Design review of the part built by this model. Coordinates are the model's own, in mm. Face numbers are marked on the shaded views. A direction names the side the tool comes from. Round coordinates to 2 decimals unless told otherwise and drop trailing zeros. Loops run counter-clockwise (first coordinate to the right, second up) from the corner with the lowest first, then second, coordinate; pieces in that order, holes last. Notation, with made-up numbers: (-34, 13.25) - (-2, 13.25) arc R19 ccw to (-2, 32.25) - close; hole circle Ø7 at (5.5, 15). An arc over 180 degrees is marked (long way). One line per question, with ' | ' between items. Start each with the question number.
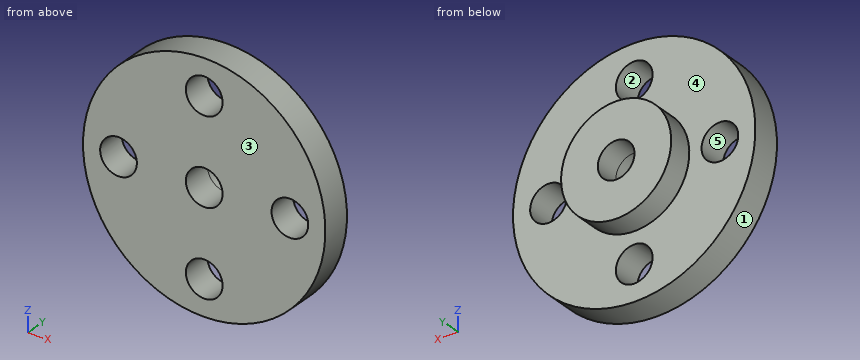
from build123d import *

# Parameters (mm, degrees)
SKETCH2_R           = 9.9
BOSS_EXTRUDE2_DEPTH = 2.45
SKETCH3_R           = 4.5
SKETCH3_R_2         = 1.5
BOSS_EXTRUDE3_DEPTH = 2.05
SKETCH5_R           = 1.5
CUT_EXTRUDE1_DEPTH  = 15.213461929
SKETCH6_R           = 1.5
CUT_EXTRUDE2_DEPTH  = 15.213461929
CIRPATTERN1_COUNT   = 4


with BuildPart() as part:
    # Sketch2 → Boss-Extrude2 (new body)
    with BuildSketch(Plane(origin=(0, 0, 0), x_dir=(1, 0, 0), z_dir=(0, 1, 0))):
        with Locations(Location((0, 0, 0), (0, 0, 270))):
            Circle(SKETCH2_R)
    extrude(amount=BOSS_EXTRUDE2_DEPTH)

    # Sketch3 → Boss-Extrude3 (add)
    with BuildSketch(Plane(origin=(0, 2.45, 0), x_dir=(1, 0, 0), z_dir=(0, 1, 0))):
        with Locations(Location((0, 0, 0), (0, 0, 270))):
            Circle(SKETCH3_R)
        with Locations(Location((0, 0, 0), (0, 0, 270))):
            Circle(SKETCH3_R_2, mode=Mode.SUBTRACT)
    extrude(amount=BOSS_EXTRUDE3_DEPTH)

    # Sketch5 → Cut-Extrude1 (cut, through all)
    with BuildSketch(Plane(origin=(0, 2.45, 0), x_dir=(1, 0, 0), z_dir=(0, 1, 0))):
        with Locations(Location((0, 0, 0), (0, 0, 270))):
            Circle(SKETCH5_R)
    extrude(amount=-CUT_EXTRUDE1_DEPTH, mode=Mode.SUBTRACT)

    # Sketch6 → Cut-Extrude2 (cut, through all)
    with BuildSketch(Plane(origin=(0, 2.45, 0), x_dir=(1, 0, 0), z_dir=(0, 1, 0))):
        with Locations(Location((7, 0, 0), (0, 0, 270))):
            Circle(SKETCH6_R)
    cut_extrude2 = extrude(amount=-CUT_EXTRUDE2_DEPTH, mode=Mode.SUBTRACT)

    # CirPattern1: Cut-Extrude2 ×4 about axis
    cirpattern1_axis = Axis((0, 0, 0), (0, 1, 0))
    for i in range(1, CIRPATTERN1_COUNT):
        add(cut_extrude2.rotate(cirpattern1_axis, i * 360 / CIRPATTERN1_COUNT), mode=Mode.SUBTRACT)


solid = part.part
1. Machinability: for the marked faces 4 and 5, which of the approach directions +Z, -Z, +X, -X, +Y, -Y give a long, thin tool a straight path to every point of the face, cutting with its end or side? Answer none if there is none.
2. Take a section at D-D, the plane x = -7. Give the boundary of the cut face in (y, z).
3. Take a section at C-C, the plane y = 2.2. Give the boundary of the cut face in (x, z), then the cut area to 3 significant figures.
4. To check wall thickness, follow line 1 along X through (y, z) = (1.45, 0); line 2 along Z through (x, y) = (0.5, 2.1); line 3 along X through (y, z) = (4, 0). State the ranges of each line that lie inside material, in increasing order.
5. Take a section at A-A, the plane x = 0. Give the boundary of the cut face in (y, z).
6. The part is to be moulded in two halves that separate along X. For the marked faces 1, 2 and 3, say which applies: pulls with the +X half, pulls with the -X half, needs draft (parallel to the pull), parting line crosses it, or undercut.
7. Clearance check with flat-ended pins moving along their axes: P1, Ø4, axis at x = 0, z = -7, coming from the +Y side; P2, Ø1, axis at x = -0.5, z = 7, coming from the +Y side; P3, Ø1, axis at x = 4, y = 1, coming from the +Z side. State where each tip first meets the part, or that it passes through.
8. Take a section at B-B, the plane z = 0. Give the boundary of the cut face in (x, y).
Answer list:
1) face 4: +Y | face 5: +Y, -Y
2) outline: (0, -7) - (2.45, -7) - (2.45, -1.5) - (0, -1.5) - close; (0, 1.5) - (2.45, 1.5) - (2.45, 7) - (0, 7) - close
3) outline: circle Ø19.8 at (0, 0); hole circle Ø3 at (-7, 0); hole circle Ø3 at (0, -7); hole circle Ø3 at (0, 0); hole circle Ø3 at (0, 7); hole circle Ø3 at (7, 0) | area: 273 mm²
4) line 1: x = -9.9 to -8.5, -5.5 to -1.5, 1.5 to 5.5, 8.5 to 9.9 | line 2: z = -9.89 to -8.41, -5.59 to -1.41, 1.41 to 5.59, 8.41 to 9.89 | line 3: x = -4.5 to -1.5, 1.5 to 4.5
5) outline: (0, -9.9) - (2.45, -9.9) - (2.45, -8.5) - (0, -8.5) - close; (0, -5.5) - (2.45, -5.5) - (2.45, -4.5) - (4.5, -4.5) - (4.5, -1.5) - (0, -1.5) - close; (0, 1.5) - (4.5, 1.5) - (4.5, 4.5) - (2.45, 4.5) - (2.45, 5.5) - (0, 5.5) - close; (0, 8.5) - (2.45, 8.5) - (2.45, 9.9) - (0, 9.9) - close
6) face 1: parting line crosses it | face 2: undercut | face 3: needs draft
7) P1: stops at y = 2.45 | P2: passes through | P3: stops at z = 9.26
8) outline: (-9.9, 0) - (-8.5, 0) - (-8.5, 2.45) - (-9.9, 2.45) - close; (-5.5, 0) - (-1.5, 0) - (-1.5, 4.5) - (-4.5, 4.5) - (-4.5, 2.45) - (-5.5, 2.45) - close; (1.5, 0) - (5.5, 0) - (5.5, 2.45) - (4.5, 2.45) - (4.5, 4.5) - (1.5, 4.5) - close; (8.5, 0) - (9.9, 0) - (9.9, 2.45) - (8.5, 2.45) - close
